```python
from build123d import *

# Parameters (mm, degrees)
F0_W     = 1828.8
F0_H     = 406.4
F1_DEPTH = 406.4
F2_T     = -19.05
F3_W     = 19.05
F3_H     = 387.35
F4_DEPTH = 368.3
F5_W     = 19.05
F5_H     = 368.3
F6_DEPTH = 25.4


with BuildPart() as f1:
    # F0 (on Front) → F1 (new body)
    with BuildSketch(Plane.XZ):
        Rectangle(F0_W, F0_H)
    extrude(amount=F1_DEPTH)

    # F2
    f2_openings = [f1.faces().sort_by_distance(p)[0] for p in [
        (0, -406.4, 0),
    ]]
    offset(amount=F2_T, openings=f2_openings)

    # F3 (on face) → F4 (join)
    with BuildSketch(Plane.XY.offset(-184.15)):
        with Locations((0, -212.725)):
            Rectangle(F3_W, F3_H)
    extrude(amount=F4_DEPTH)

    # F5 (on face) → F6 (cut)
    with BuildSketch(Plane.XZ.offset(406.4)):
        Rectangle(F5_W, F5_H)
    extrude(amount=-F6_DEPTH, mode=Mode.SUBTRACT)


solid = f1.part
```
Can you work these out from the model? Positions are in its coordinate system, mm. A direction names the side the tool comes from. Give positions to 0.01 mm unless a question says otherwise; leave off trailing zeros. Loops run counter-clockwise (first coordinate to the right, second up) from the corner with the lowest first, then second, coordinate; pieces in that order, holes last. Notation, with made-up numbers: M -36,0 L 9,0 A24 ccw 9,14 Z; hole C 55.25,3 d7. An arc over 180 degrees is marked long. Use one line per item in the form item = value. Start each with the question number.
(1) Thinking about a two-plate mould opening in X: for faces 1 (the flat face through (914.4, -200, -3)), 2 (the flat face through (-4, -406.4, 197)), 3 (the flat face through (-13, -210, -184.15)), which applies, released by +X, released by -X, zero draft, split by the parting line, or undercut?
(2) I'm going to push a flat-ended pin straight in: P1, Ø9.5, axis at x = -3, z = 43.5, coming from the -Y side. Where does the tip first touch, or does it pass through?
(3) On a 3-axis mill with a long thin cutter (end or side, diameter ignored), from which of +Z, -Z, +X, -X, +Y, -Y can I reach the whole of each face in a straight line? I mean faces 4 (the flat face through (-914.4, -200, -3)), 5 (the flat face through (895.35, -210, -3)). Say none if no direction works.
(4) I want a section at C-C, the plane x = 627. Write out the boundary of the cut face in (y, z), and give its area (3 significant figures).
(5) I want a section at A-A, the plane y = -229. Write out the boundary of the cut face in (x, z) (3 decimals).
(6) Please list where these lines run through material, in increasing order: line 1 (X direction, y = -207, z = 167.5) (3 decimals); line 2 (Z direction, x = 652.5, y = -136.5).
(7) I want a section at B-B, the plane z = 152. Write out the boundary of the cut face in (x, y) (3 decimals).
Worked out:
q1.face_1 = released by +X
q1.face_2 = zero draft
q1.face_3 = undercut
q2.P1 = -381
q3.face_4 = +Z, -Z, -X, +Y, -Y
q3.face_5 = -Y
q4.outline = M -406.4,-203.2 L 0,-203.2 L 0,203.2 L -406.4,203.2 L -406.4,184.15 L -19.05,184.15 L -19.05,-184.15 L -406.4,-184.15 Z
q4.area = 22,500 mm²
q5.outline = M -914.4,-203.2 L 914.4,-203.2 L 914.4,203.2 L -914.4,203.2 Z; hole M -895.35,-184.15 L -9.525,-184.15 L -9.525,184.15 L -895.35,184.15 Z; hole M 9.525,-184.15 L 895.35,-184.15 L 895.35,184.15 L 9.525,184.15 Z
q6.line_1 = -914.4 to -895.35, -9.525 to 9.525, 895.35 to 914.4
q6.line_2 = -203.2 to -184.15, 184.15 to 203.2
q7.outline = M -914.4,-406.4 L -895.35,-406.4 L -895.35,-19.05 L -9.525,-19.05 L -9.525,-381 L 9.525,-381 L 9.525,-19.05 L 895.35,-19.05 L 895.35,-406.4 L 914.4,-406.4 L 914.4,0 L -914.4,0 Z
